from build123d import *

# Parameters (mm, degrees)
SKICA1_W                = 57
SKICA1_H                = 67
SKICA1_R                = 2
P_IDAT_VYSUNUT_M1_DEPTH = 3
P_IDAT_VYSUNUT_M2_DEPTH = 1


with BuildPart() as part:
    # Skica1 → Přidat vysunutím1 (new body)
    with BuildSketch(Plane.XY):
        with Locations((28.5, 33.5)):
            Rectangle(SKICA1_W, SKICA1_H)
        with Locations((3.5, 62.35016579)):
            Circle(SKICA1_R, mode=Mode.SUBTRACT)
        with Locations((53.5, 62.35016579)):
            Circle(SKICA1_R, mode=Mode.SUBTRACT)
        with Locations((53.5, 3.5)):
            Circle(SKICA1_R, mode=Mode.SUBTRACT)
        with Locations((3.5, 3.5)):
            Circle(SKICA1_R, mode=Mode.SUBTRACT)
    extrude(amount=P_IDAT_VYSUNUT_M1_DEPTH)

    # Skica2 → Přidat vysunutím2 (add)
    with BuildSketch(Plane(origin=(0, 0, 0), x_dir=(-1, 0, 0), z_dir=(0, 0, -1))):
        Polygon((-41.396588298, 31.388427372), (-41.396588298, 33.183299167), (-23.447870349, 33.183299167), (-23.447870349, 40.87560686), (-21.396588298, 40.87560686), (-21.396588298, 31.388427372), align=None)
    extrude(amount=P_IDAT_VYSUNUT_M2_DEPTH)


solid = part.part
Work out the finished part from the listing and answer in its coordinate system (mm). Coordinates: 2 decimals unless noted, no trailing zeros. Order: outer loops, then holes, each group sorted by start corner. A loop starts at its lowest first (then second) coordinate and runs counter-clockwise, first axis right, second up. Notation, with made-up numbers: (55.25, 68.5) - (97.25, 68.5) arc R33 ccw to (97.25, 106.5) - close; hole circle Ø9 at (-20.75, 10). An arc over 180 degrees is marked (long way). Put each result on its own line as item: value. Start each with the question number.
1) Find the intervals of material crossed by line 1 (Y direction, x = 53.5, z = 0.6); line 2 (Y direction, x = 5, z = 1.3); line 3 (Z direction, x = 34, y = 17), in increasing order. Write a range as from..to.
2) Find section C-C (x = 53.5). Give the vertices of the cut face in (y, z), plus the area to 3 significant figures.
3) For a pull along X with two mould halves and no side action, classify faces 1 (the flat face through (57, 33, 1)), 2 (the cylindrical face through (1.502, 3.588, 1.479)), 3 (the flat face through (28, 34, 3)) as released by +X, released by -X, zero draft, split by the parting line, or undercut.
4) Flat-ended cylindrical pins translate along their axes: pin 1 (0.8 mm diameter, centred on y = 37.5, z = -0.5, fed in from +X); pin 2 (0.8 mm diameter, centred on x = 22.5, z = -0.5, fed in from +Y); pin 3 (6.5 mm diameter, centred on x = 3.5, y = 3.5, fed in from -Z). Find the tip coordinate at first contact, or state that the pin passes through.
5) Find section B-B (x = 28.5). Give the vertices of the cut face in (y, z).
6) Find section A-A (y = 3.5). Give the vertices of the cut face in (x, z), plus the area to 3 significant figures.
Results list:
1. line 1: y = 0..1.5, 5.5..60.35, 64.35..67
1. line 2: y = 0..2.18, 4.82..61.03, 63.67..67
1. line 3: z = 0..3
2. outline: (0, 0) - (1.5, 0) - (1.5, 3) - (0, 3) - close; (5.5, 0) - (60.35, 0) - (60.35, 3) - (5.5, 3) - close; (64.35, 0) - (67, 0) - (67, 3) - (64.35, 3) - close
2. area: 177 mm^2
3. face 1: released by +X
3. face 2: undercut
3. face 3: zero draft
4. pin 1: stops at x = 23.45
4. pin 2: stops at y = 40.88
4. pin 3: stops at z = 0
5. outline: (0, 0) - (31.39, 0) - (31.39, -1) - (33.18, -1) - (33.18, 0) - (67, 0) - (67, 3) - (0, 3) - close
6. outline: (0, 0) - (1.5, 0) - (1.5, 3) - (0, 3) - close; (5.5, 0) - (51.5, 0) - (51.5, 3) - (5.5, 3) - close; (55.5, 0) - (57, 0) - (57, 3) - (55.5, 3) - close
6. area: 147 mm^2
